from build123d import *

# Parameters (mm, degrees)
BOSS_EXTRUDE1_DEPTH = 12
SKETCH4_R           = 12.5
SKETCH4_R_2         = 2
CUT_EXTRUDE1_DEPTH  = 20


with BuildPart() as part:
    # Sketch2 → Boss-Extrude1 (new body)
    with BuildSketch(Plane(origin=(0, 0, 0), x_dir=(1, 0, 0), z_dir=(0, 1, 0))):
        Polygon((-318.206861599, 87.608284791), (-18.206861599, 0), (31.793138401, 0), (331.793138401, 87.608284791), (331.793138401, 117.608284791), (301.793138401, 117.608284791), (31.793138401, 70), (-18.206861599, 70), (-288.206861599, 117.608284791), (-318.206861599, 117.608284791), align=None)
    extrude(amount=BOSS_EXTRUDE1_DEPTH)

    # Sketch4 → Cut-Extrude1 (cut)
    with BuildSketch(Plane(origin=(0, 12, 0), x_dir=(1, 0, 0), z_dir=(0, 1, 0))):
        with Locations((6.793138401, 35)):
            Circle(SKETCH4_R)
        with Locations((6.793138401, 53.5)):
            Circle(SKETCH4_R_2)
        with Locations((22.814608371, 44.25)):
            Circle(SKETCH4_R_2)
        with Locations((22.814608371, 25.75)):
            Circle(SKETCH4_R_2)
        with Locations((6.793138401, 16.5)):
            Circle(SKETCH4_R_2)
        with Locations((-9.228331569, 25.75)):
            Circle(SKETCH4_R_2)
        with Locations((-9.228331569, 44.25)):
            Circle(SKETCH4_R_2)
    extrude(amount=-CUT_EXTRUDE1_DEPTH, mode=Mode.SUBTRACT)


solid = part.part
Build history of the part. All positions in model axes, mm. A direction names the side the tool comes from. Give positions to 0.01 mm unless a question says otherwise; leave off trailing zeros. Order: outer loops, then holes, each group sorted by start corner. A loop starts at its lowest first (then second) coordinate and runs counter-clockwise, first axis right, second up. Notation, with made-up numbers: M 88,72 L 120,72 A30 cw 120,109 Z; hole C 13,84 d7. An arc over 180 degrees is marked long. Put each result on its own line as item: value.
Item 1: Slice it at C-C, the plane z = -35. Write the cut outline in (x, y), plus the area to 3 significant figures.
From the geometry:
outline: M -138.06,0 L -5.71,0 L -5.71,12 L -138.06,12 Z; M 19.29,0 L 151.64,0 L 151.64,12 L 19.29,12 Z
area: 3,180 mm2
Item 2: 3-axis set-ups, long thin cutter, end or side, ignore diameter. For faces 4 (the flat face through (317, 6, -117.608)), 5 (the flat face through (168.683, 5.916, -94.137)): which of +Z, -Z, +X, -X, +Y, -Y reach the whole face in a straight line?
From the geometry:
face 4: -Z, +X, -X, +Y, -Y
face 5: -Z, +Y, -Y
Item 3: Two-plate mould, pull along X, no slides. Class faces 1 (the flat face through (2, 12, -60)), 2 (the flat face through (-151.32, 5.92, -93.47)), 3 (the flat face through (-170.31, 5.92, -44.42)): +X half, -X half, draft (parallel to the pull), parting line (faces both ways), or undercut.
From the geometry:
face 1: draft
face 2: undercut
face 3: -X half
Item 4: Probe line 1 (Z direction, x = -9, y = 3); line 2 (Z direction, x = 296.5, y = 1.25); line 3 (Z direction, x = 85, y = 5.25). List the from-to ranges inside material, lowest first. Write a range as [from, to].
From the geometry:
line 1: z = [-70, -46.24], [-42.26, -27.74], [-23.76, 0]
line 2: z = [-116.67, -77.3]
line 3: z = [-79.38, -15.54]
Item 5: Slice it at D-D, the plane x = -253. Write the cut outline in (y, z).
From the geometry:
outline: M 0,-111.4 L 12,-111.4 L 12,-68.57 L 0,-68.57 Z
Item 6: Flat gauge pins, fed straight in: pin 1 Ø6.5 at (x, z) = (22.81, -25.75) entering from +Y; pin 2 Ø3 at (x, y) = (123, 9.5) entering from -Z; pin 3 Ø3.5 at (x, y) = (1, 3.5) entering from -Z. Where does each tip first touch, or does it go through?
From the geometry:
pin 1: stops at y = 12
pin 2: stops at z = -86.35
pin 3: stops at z = -70
Item 7: Slice it at A-A, the plane z = -96.5. Write the cut outline in (x, y), plus the area to 3 significant figures.
From the geometry:
outline: M -318.21,0 L -168.5,0 L -168.5,12 L -318.21,12 Z; M 182.08,0 L 331.79,0 L 331.79,12 L 182.08,12 Z
area: 3,590 mm2
Item 8: Slice it at B-B, the plane y = 9. Write the cut outline in (x, z), plus the area to 3 significant figures.
From the geometry:
outline: M -318.21,-117.61 L -288.21,-117.61 L -18.21,-70 L 31.79,-70 L 301.79,-117.61 L 331.79,-117.61 L 331.79,-87.61 L 31.79,0 L -18.21,0 L -318.21,-87.61 Z; hole C -9.23,-44.25 d4; hole C -9.23,-25.75 d4; hole C 6.79,-35 d25; hole C 6.79,-53.5 d4; hole C 6.79,-16.5 d4; hole C 22.81,-44.25 d4; hole C 22.81,-25.75 d4
area: 34,400 mm2
